from build123d import *

# Parameters (mm, degrees)
SKETCH_1_W          = 45.5
SKETCH_1_H          = 21.5
EXTRUDE_1_DEPTH     = 1
SKETCH_2_W          = 6
SKETCH_2_H          = 15
EXTRUDE_2_DEPTH     = 2
SKETCH_3_R          = 8.05
CUT_EXTRUDE_1_DEPTH = 30.599408778
CUT_EXTRUDE_2_DEPTH = 30.599408778
SKETCH_5_R          = 1.6
CUT_EXTRUDE_3_DEPTH = 38.320403267
SKETCH_6_R          = 8.05
EXTRUDE_3_DEPTH     = 1


with BuildPart() as part:
    # 草圖1 → 填料-伸長1 (new body)
    with BuildSketch(Plane(origin=(0, 0, 0), x_dir=(1, 0, 0), z_dir=(0, 1, 0))):
        Rectangle(SKETCH_1_W, SKETCH_1_H)
    extrude(amount=EXTRUDE_1_DEPTH)

    # 草圖2 → 填料-伸長2 (add)
    with BuildSketch(Plane.XY.offset(10.75)):
        with Locations((-19.75, 7.5)):
            Rectangle(SKETCH_2_W, SKETCH_2_H)
        with Locations((19.75, 7.5)):
            Rectangle(SKETCH_2_W, SKETCH_2_H)
    extrude_2 = extrude(amount=EXTRUDE_2_DEPTH)

    # 鏡射1: 填料-伸長2 across plane
    add(extrude_2.mirror(Plane.XY))

    # 草圖3 → 除料-伸長1 (cut, through all)
    with BuildSketch(Plane(origin=(0, 1, 0), x_dir=(1, 0, 0), z_dir=(0, 1, 0))):
        with Locations(Location((-12.94, -0.6, 0), (0, 0, 270))):
            Circle(SKETCH_3_R)
        with Locations(Location((12.94, -0.6, 0), (0, 0, 270))):
            Circle(SKETCH_3_R)
    extrude(amount=-CUT_EXTRUDE_1_DEPTH, mode=Mode.SUBTRACT)

    # 草圖4 → 除料-伸長2 (cut, through all)
    with BuildSketch(Plane(origin=(0, 1, 0), x_dir=(1, 0, 0), z_dir=(0, 1, 0))):
        with BuildLine():
            Line((-3.25, -5.95), (3.25, -5.95))
            ThreePointArc((3.25, -5.95), (5, -7.7), (3.25, -9.45))
            Line((3.25, -9.45), (-3.25, -9.45))
            ThreePointArc((-3.25, -9.45), (-5, -7.7), (-3.25, -5.95))
        make_face()
    extrude(amount=-CUT_EXTRUDE_2_DEPTH, mode=Mode.SUBTRACT)

    # 草圖5 → 除料-伸長3 (cut, through all)
    with BuildSketch(Plane(origin=(0, 0, -12.75), x_dir=(-1, 0, 0), z_dir=(0, 0, -1))):
        with Locations((19.75, 9)):
            Circle(SKETCH_5_R)
        with Locations((-19.75, 9)):
            Circle(SKETCH_5_R)
    extrude(amount=-CUT_EXTRUDE_3_DEPTH, mode=Mode.SUBTRACT)

    # 草圖6 → 填料-伸長3 (add)
    with BuildSketch(Plane.XZ):
        Polygon((-22.75, 12.75), (-22.75, -12.75), (-16.75, -12.75), (-16.75, -10.75), (16.75, -10.75), (16.75, -12.75), (22.75, -12.75), (22.75, 12.75), (16.75, 12.75), (16.75, 10.75), (-16.75, 10.75), (-16.75, 12.75), align=None)
        with Locations(Location((-12.94, 0.6, 0), (0, 0, 90))):
            Circle(SKETCH_6_R, mode=Mode.SUBTRACT)
        with Locations(Location((12.94, 0.6, 0), (0, 0, 90))):
            Circle(SKETCH_6_R, mode=Mode.SUBTRACT)
        with BuildLine():
            Line((3.25, 5.95), (-3.25, 5.95))
            ThreePointArc((-3.25, 5.95), (-5, 7.7), (-3.25, 9.45))
            Line((-3.25, 9.45), (3.25, 9.45))
            ThreePointArc((3.25, 9.45), (5, 7.7), (3.25, 5.95))
        make_face(mode=Mode.SUBTRACT)
    extrude(amount=EXTRUDE_3_DEPTH)


solid = part.part
Can you work these out from the model? Positions are in its coordinate system, mm. A direction names the side the tool comes from. Coordinates: 2 decimals unless noted, no trailing zeros. Write each loop counter-clockwise with the first axis right and the second up, starting at its lowest first coordinate (ties: lowest second). Pieces come first, ordered by that corner, then holes. Notation, with made-up numbers: (-16, 85.25) -> (6, 85.25) arc R6 cw to (6, 90.25) -> close; hole circle Ø7 at (25, 47.25). An arc over 180 degrees is marked (long way). Write each question's results on one line, items separated by ' | '. Start each with the question number.
Item 1: Thinking about a two-plate mould opening in X: for faces 1 (the flat face through (0, 0, 5.95)), 2 (the flat face through (22.75, 0.5, 0.9)), 3 (the cylindrical face through (-19.4, 7.44, 11.74)), 4 (the flat face through (20, 7, -12.75)), which applies, released by +X, released by -X, zero draft, split by the parting line, or undercut?
Item 2: If we section it at B-B, the plane z = 0.6: Write out the boundary of the cut face in (x, y), and give its area (3 significant figures).
Item 3: On a 3-axis mill with a long thin cutter (end or side, diameter ignored), from which of +Z, -Z, +X, -X, +Y, -Y can I reach the whole of each face in a straight line? I mean faces 5 (the cylindrical face through (-5, 0, 7.7)), 6 (the flat face through (20, 7, 12.75)), 7 (the flat face through (-20, 7, 10.75)). Say none if no direction works.
Item 4: Please list where these lines run through material, in increasing order: probe 1 along X at (y, z) = (-0.1, 0.6); probe 2 along Z at (x, y) = (-18, 10.25); probe 3 along Y at (x, z) = (-19.75, 11.8).
Item 5: If we section it at C-C, the plane y = 6: Write out the boundary of the cut face in (x, z).
Item 6: I'm going to push flat-ended pins straight in: P1, Ø1.6, axis at x = 1, y = 0.5, coming from the +Z side; P2, Ø6.5, axis at x = 11, z = -4.5, coming from the +Y side; P3, Ø2.5, axis at x = 19.75, y = 9, coming from the +Z side; P4, Ø5, axis at y = 2.5, z = -8, coming from the -X side. Where does each tip first touch, or does it pass through?
Item 7: If we section it at A-A, the plane x = -12.94: Write out the boundary of the cut face in (y, z), and give its area (3 significant figures).
Item 8: If we section it at D-D, the plane y = 9: Count the separate pieces of the cut face and the enclosed holes in it, and give its area (3 significant figures).
Answer block:
1) face 1: undercut | face 2: released by +X | face 3: undercut | face 4: zero draft
2) outline: (-22.75, -1) -> (-20.99, -1) -> (-20.99, 1) -> (-22.75, 1) -> close; (-4.89, -1) -> (4.89, -1) -> (4.89, 1) -> (-4.89, 1) -> close; (20.99, -1) -> (22.75, -1) -> (22.75, 1) -> (20.99, 1) -> close | area: 26.6 mm²
3) face 5: +Y, -Y | face 6: +Z, +X, -X, +Y, -Y | face 7: +X, -X, +Y
4) probe 1: -22.75 to -20.99, -4.89 to 4.89, 20.99 to 22.75 | probe 2: -12.75 to -10.75, 10.75 to 12.75 | probe 3: -1 to 7.4, 10.6 to 15
5) outline: (-22.75, -12.75) -> (-16.75, -12.75) -> (-16.75, -10.75) -> (-22.75, -10.75) -> close; (-22.75, 10.75) -> (-16.75, 10.75) -> (-16.75, 12.75) -> (-22.75, 12.75) -> close; (16.75, -12.75) -> (22.75, -12.75) -> (22.75, -10.75) -> (16.75, -10.75) -> close; (16.75, 10.75) -> (22.75, 10.75) -> (22.75, 12.75) -> (16.75, 12.75) -> close
6) P1: z = 10.75 | P2: y = 1 | P3: through | P4: x = -22.75
7) outline: (-1, -10.75) -> (1, -10.75) -> (1, -7.45) -> (-1, -7.45) -> close; (-1, 8.65) -> (1, 8.65) -> (1, 10.75) -> (-1, 10.75) -> close | area: 10.8 mm²
8) separate pieces: 8 | enclosed holes: 0 | area: 22.4 mm²
